Part model, mm, in its own coordinate system. Face numbers are marked on the shaded views. A direction names the side the tool comes from. Coordinates: 2 decimals unless noted, no trailing zeros. Loops run counter-clockwise (first coordinate to the right, second up) from the corner with the lowest first, then second, coordinate; pieces in that order, holes last.
```python
from build123d import *

# Parameters (mm, degrees)
F1_DEPTH = 15.7734
F3_D     = 20.32
F5_DEPTH = 20.828
F6_DEPTH = 16.002
F8_R     = 3.302
F9_DEPTH = 39.37


with BuildPart() as f1:
    # F0 (on Top) → F1 (new body)
    with BuildSketch(Plane.XY):
        with BuildLine():
            Line((27.2614864262, -32.5740104774), (-27.2614864262, -32.5740104774))
            Line((-27.2614864262, -32.5740104774), (-19.05, -86.5490104774))
            ThreePointArc((-19.05, -86.5490104774), (0, -103.6707926836), (19.05, -86.5490104774))
            Line((19.05, -86.5490104774), (27.2614864262, -32.5740104774))
        make_face()
    extrude(amount=F1_DEPTH)

    # F3 (through all)
    with Locations(Plane.XY.offset(15.7734)):
        with Locations((0, -89.5141884685)):
            Hole(F3_D / 2)

    # F4 (on face) → F5 (join)
    with BuildSketch(Plane.XY.offset(15.7734)):
        with BuildLine():
            ThreePointArc((27.2197921324, -32.8480716384), (29.2060026188, -26.8297481215), (29.8781534287, -20.5278862268))
            ThreePointArc((29.8781534287, -20.5278862268), (-6.3018618947, 8.678116392), (-27.2197921324, -32.8480716384))
            Line((-27.2197921324, -32.8480716384), (-27.2614864262, -32.5740104774))
            Line((-27.2614864262, -32.5740104774), (-16.4541315907, -32.5740104774))
            ThreePointArc((-16.4541315907, -32.5740104774), (0.0596223919, -1.2802406646), (16.5733763745, -32.5740104774))
            Line((16.5733763745, -32.5740104774), (27.2614864262, -32.5740104774))
            Line((27.2614864262, -32.5740104774), (27.2197921324, -32.8480716384))
        make_face()
        with BuildLine():
            Line((-27.2614864262, -32.5740104774), (-27.2197921324, -32.8480716384))
            ThreePointArc((-27.2197921324, -32.8480716384), (0, -50.4060396555), (27.2197921324, -32.8480716384))
            Line((27.2197921324, -32.8480716384), (27.2614864262, -32.5740104774))
            Line((27.2614864262, -32.5740104774), (16.5733763745, -32.5740104774))
            Line((16.5733763745, -32.5740104774), (-16.4541315907, -32.5740104774))
            Line((-16.4541315907, -32.5740104774), (-27.2614864262, -32.5740104774))
        make_face()
    extrude(amount=F5_DEPTH)

    # F6 (add): a face of the model
    f6_faces = [f1.faces().sort_by_distance(p)[0] for p in [
        (-21.8578090084, -31.8424699105, 15.7734),
    ]]
    extrude(f6_faces, amount=F6_DEPTH)

    # F8
    f8_edges = [f1.edges().sort_by_distance(p)[0] for p in [
        (-29.878153, -20.527886, 36.6014),
    ]]
    fillet(f8_edges, radius=F8_R)

    # F7 (on face) → F9 (cut)
    with BuildSketch(Plane(origin=(0, 0, 0), x_dir=(1, 0, 0), z_dir=(0, 0, -1))):
        with BuildLine():
            Line((-5.2386547938, 43.5478799045), (-5.2386547938, 39.4042106377))
            ThreePointArc((-5.2386547938, 39.4042106377), (-11.348132673, 36.8129879511), (-16.4541315907, 32.5740104774))
            Line((-16.4541315907, 32.5740104774), (16.5733763745, 32.5740104774))
            ThreePointArc((16.5733763745, 32.5740104774), (11.4254150287, 36.8533502525), (5.2473828261, 39.43136752))
            Line((5.2473828261, 39.43136752), (5.2473828261, 43.5478799045))
            Line((5.2473828261, 43.5478799045), (-5.2386547938, 43.5478799045))
        make_face()
    extrude(amount=-F9_DEPTH, mode=Mode.SUBTRACT)


solid = f1.part
```
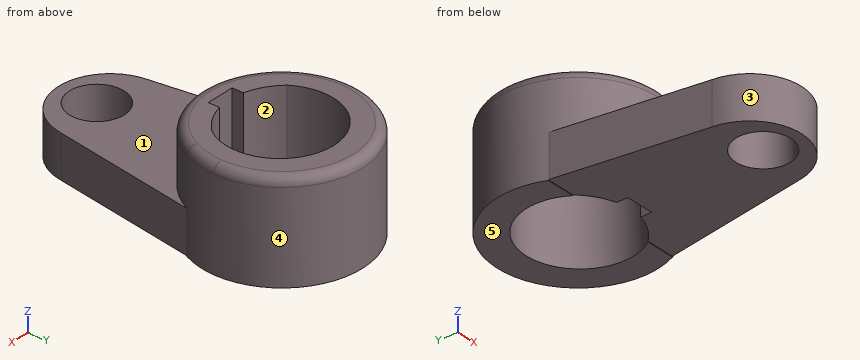
Q1. Probe line 1 (Y direction, x = 4, z = 4); line 2 (Y direction, x = -6.5, z = 2); line 3 (Z direction, x = -18.5, y = -63). List the from-to ranges inside material, lowest first.
Q2. Tool access for the marked faces 4 and 5: list every direction of +Z, -Z, +X, -X, +Y, -Y with a clear straight run to the whole face (end or side of a thin tool).
Q3. Mould opens along X. For the marked faces 1, 2 and 3 say: released by +X, released by -X, zero draft, split by the parting line, or undercut.
Q4. Drop flat-ended pins along their axis: P1, Ø2, axis at x = 14, z = 16.5, coming from the -Y side; P2, Ø2, axis at y = -41, z = 24.5, coming from the -X side; P3, Ø24, axis at x = 0.06, y = -21.28, coming from the +Z side; P4, Ø6, axis at x = -8.5, z = 30, coming from the +Y side. Give the stop position or say it passes through.
Q5. Saw through at B-B (z = 13). List the corners of the cut face in (x, y), plus the area to 3 significant figures.
Q6. Saw through at C-C (x = -3). Count the separate pieces of the cut face and the enclosed holes in it, plus the area to 3 significant figures.
Q7. Saw through at A-A (z = 20). List the corners of the cut face in (x, y), plus the area to 3 significant figures.
Checked values:
1. line 1: y = -103.25 to -98.85, -80.17 to -43.55, -1.67 to 9.08
1. line 2: y = -102.53 to -97.32, -81.71 to -39.04, -2.39 to 8.63
1. line 3: z = 0 to 15.77
2. face 4: +Z
2. face 5: -Z, +X, -X, +Y, -Y
3. face 1: zero draft
3. face 2: undercut
3. face 3: split by the parting line
4. P1: stops at y = -98.29
4. P2: stops at x = -22.66
4. P3: passes through
4. P4: stops at y = 8.84
5. outline: (-27.22, -32.85) - (-19.05, -86.55) arc R19.16 ccw to (19.05, -86.55) - (27.22, -32.85) arc R29.88 ccw (long way) to start; hole (-16.45, -32.57) arc R22.83 ccw to (-5.24, -39.4) - (-5.24, -43.55) - (5.25, -43.55) - (5.25, -39.43) arc R22.53 ccw to (16.57, -32.57) arc R20 ccw (long way) to start; hole circle Ø20.32 at (0, -89.51)
5. area: 3,510 mm2
6. separate pieces: 3
6. enclosed holes: 0
6. area: 1,170 mm2
7. outline: circle Ø59.76 at (0, -20.53); hole (-16.45, -32.57) arc R22.83 ccw to (-5.24, -39.4) - (-5.24, -43.55) - (5.25, -43.55) - (5.25, -39.43) arc R22.53 ccw to (16.57, -32.57) arc R20 ccw (long way) to start
7. area: 1,540 mm2
